Design review of the part built by this model. Coordinates are the model's own, in mm. A direction names the side the tool comes from. Coordinates: 2 decimals unless noted, no trailing zeros. Write each loop counter-clockwise with the first axis right and the second up, starting at its lowest first coordinate (ties: lowest second). Pieces come first, ordered by that corner, then holes.
Q1. For probe 1 along X at (y, z) = (10, 10.5); probe 2 along Y at (x, z) = (70, 4); probe 3 along Z at (x, y) = (27.5, -21.5), list the stretches that pass through material, from the lowest coordinate up.
Q2. Mouldability with a two-part tool opening along Y and no side actions: class faces 3 (the flat face through (-1, 22, -1)), 4 (the cylindrical face through (40, -20, 0)) as pulls with the +Y half, pulls with the -Y half, needs draft (parallel to the pull), parting line crosses it, or undercut.
Q3. Insertion check: pin 1 (0.5 mm diameter, centred on x = 27.5, y = -13, fed in from -Z); pin 2 (1.2 mm diameter, centred on x = 71, y = -13.5, fed in from +Z); pin 3 (5 mm diameter, centred on x = 45, y = -6.5, fed in from +Z); pin 4 (0.5 mm diameter, centred on x = 8, y = -13.5, fed in from +Z). Each pin has a flat end and moves straight along its axis. Give the tip position at first contact, or say it passes through.
Q4. Take a section at D-D (y = 14). Give the boundary of the cut face in (x, z).
Q5. Take a section at A-A (y = -3.5). Give the boundary of the cut face in (x, z).
Q6. Take a section at B-B (x = 5). State how many separate pieces and enclosed holes the cut face has, and give its area (3 significant figures).
Q7. Take a section at C-C (z = 22.5). Give the boundary of the cut face in (x, y).
Q8. Machinability: for faces 1 (the flat face through (30, -20, 4)), 2 (the flat face through (78.33, 23.87, 41.13)), which of the approach directions +Z, -Z, +X, -X, +Y, -Y give a long, thin tool a straight path to every point of the face, cutting with its end or side? Answer none if there is none.
```python
from build123d import *

# Parameters (mm, degrees)
BOSS_EXTRUDE1_DEPTH     = 80
CUT_EXTRUDE1_DEPTH      = 116.337274212
CUT_EXTRUDE1_DEPTH_BACK = 116.337274212
SKETCH2_W               = 76
SKETCH2_H               = 61.532163543
SKETCH3_W               = 18
SKETCH3_H               = 14.744736797
CUT_EXTRUDE2_DEPTH      = 20
BOSS_EXTRUDE2_DEPTH     = 1
BOSS_EXTRUDE3_START     = -81
BOSS_EXTRUDE3_DEPTH     = 1


with BuildPart() as part:
    # Sketch1 → Boss-Extrude1 (new body)
    with BuildSketch(Plane(origin=(0, 0, 0), x_dir=(0, 0, -1), z_dir=(1, 0, 0))):
        with BuildLine():
            Line((-17.20219293, -12.045105163), (-63.088307838, 53.48705838))
            Line((-63.088307838, 53.48705838), (-62.269155794, 54.060634816))
            Line((-62.269155794, 54.060634816), (-16.383040886, -11.471528727))
            ThreePointArc((-16.383040886, -11.471528727), (0, -20), (16.383040886, -11.471528727))
            Line((16.383040886, -11.471528727), (62.269155794, 54.060634816))
            Line((62.269155794, 54.060634816), (63.088307838, 53.48705838))
            Line((63.088307838, 53.48705838), (17.20219293, -12.045105163))
            ThreePointArc((17.20219293, -12.045105163), (0, -21), (-17.20219293, -12.045105163))
        make_face()
        with BuildLine():
            ThreePointArc((7.788873039, -19.5021398), (0, -21), (-7.788873039, -19.5021398))
            ThreePointArc((-7.788873039, -19.5021398), (-2.130530499, -24.056165822), (0, -31))
            ThreePointArc((0, -31), (2.130530499, -24.056165822), (7.788873039, -19.5021398))
        make_face()
    extrude(amount=BOSS_EXTRUDE1_DEPTH)

    # Sketch2 → Cut-Extrude1 (cut, two sides: drawn at the far end of the back side and taken through both)
    with BuildSketch(Plane.XY.offset(-CUT_EXTRUDE1_DEPTH_BACK)):
        with Locations((40, 20.720976608)):
            Rectangle(SKETCH2_W, SKETCH2_H)
    extrude(amount=CUT_EXTRUDE1_DEPTH + CUT_EXTRUDE1_DEPTH_BACK, mode=Mode.SUBTRACT)

    # Sketch3 → Cut-Extrude2 (cut)
    with BuildSketch(Plane(origin=(0, 0, 0), x_dir=(1, 0, 0), z_dir=(0, 1, 0))):
        with Locations((10, -8.191520442)):
            Rectangle(SKETCH3_W, SKETCH3_H)
        with Locations((10, 8.191520442)):
            Rectangle(SKETCH3_W, SKETCH3_H)
        with Locations((30, 8.191520442)):
            Rectangle(SKETCH3_W, SKETCH3_H)
        with Locations((30, -8.191520442)):
            Rectangle(SKETCH3_W, SKETCH3_H)
        with Locations((50, -8.191520442)):
            Rectangle(SKETCH3_W, SKETCH3_H)
        with Locations((50, 8.191520442)):
            Rectangle(SKETCH3_W, SKETCH3_H)
        with Locations((70, -8.191520442)):
            Rectangle(SKETCH3_W, SKETCH3_H)
        with Locations((70, 8.191520442)):
            Rectangle(SKETCH3_W, SKETCH3_H)
    extrude(amount=-CUT_EXTRUDE2_DEPTH, mode=Mode.SUBTRACT)

    # Sketch4 → Boss-Extrude2 (add)
    with BuildSketch(Plane(origin=(80, 0, 0), x_dir=(0, 0, -1), z_dir=(1, 0, 0))):
        with BuildLine():
            Line((-62.269155794, 54.060634816), (62.269155794, 54.060634816))
            Line((62.269155794, 54.060634816), (16.383040886, -11.471528727))
            ThreePointArc((16.383040886, -11.471528727), (0, -20), (-16.383040886, -11.471528727))
            Line((-16.383040886, -11.471528727), (-62.269155794, 54.060634816))
        make_face()
        with BuildLine():
            Line((-62.269155794, 54.060634816), (-63.088307838, 53.48705838))
            Line((-63.088307838, 53.48705838), (-17.20219293, -12.045105163))
            ThreePointArc((-17.20219293, -12.045105163), (-13.03994578, -16.460857026), (-7.788873039, -19.5021398))
            ThreePointArc((-7.788873039, -19.5021398), (-2.130530499, -24.056165822), (0, -31))
            ThreePointArc((0, -31), (2.130530499, -24.056165822), (7.788873039, -19.5021398))
            ThreePointArc((7.788873039, -19.5021398), (13.03994578, -16.460857026), (17.20219293, -12.045105163))
            Line((17.20219293, -12.045105163), (63.088307838, 53.48705838))
            Line((63.088307838, 53.48705838), (62.269155794, 54.060634816))
            Line((62.269155794, 54.060634816), (16.383040886, -11.471528727))
            ThreePointArc((16.383040886, -11.471528727), (0, -20), (-16.383040886, -11.471528727))
            Line((-16.383040886, -11.471528727), (-62.269155794, 54.060634816))
        make_face()
    extrude(amount=BOSS_EXTRUDE2_DEPTH)

    # Sketch4<3> → Boss-Extrude3 (add)
    with BuildSketch(Plane(origin=(80, 0, 0), x_dir=(0, 0, -1), z_dir=(1, 0, 0)).offset(BOSS_EXTRUDE3_START)):
        with BuildLine():
            Line((-62.269155794, 54.060634816), (62.269155794, 54.060634816))
            Line((62.269155794, 54.060634816), (16.383040886, -11.471528727))
            ThreePointArc((16.383040886, -11.471528727), (0, -20), (-16.383040886, -11.471528727))
            Line((-16.383040886, -11.471528727), (-62.269155794, 54.060634816))
        make_face()
        with BuildLine():
            Line((-62.269155794, 54.060634816), (-63.088307838, 53.48705838))
            Line((-63.088307838, 53.48705838), (-17.20219293, -12.045105163))
            ThreePointArc((-17.20219293, -12.045105163), (-13.03994578, -16.460857026), (-7.788873039, -19.5021398))
            ThreePointArc((-7.788873039, -19.5021398), (-2.130530499, -24.056165822), (0, -31))
            ThreePointArc((0, -31), (2.130530499, -24.056165822), (7.788873039, -19.5021398))
            ThreePointArc((7.788873039, -19.5021398), (13.03994578, -16.460857026), (17.20219293, -12.045105163))
            Line((17.20219293, -12.045105163), (63.088307838, 53.48705838))
            Line((63.088307838, 53.48705838), (62.269155794, 54.060634816))
            Line((62.269155794, 54.060634816), (16.383040886, -11.471528727))
            ThreePointArc((16.383040886, -11.471528727), (0, -20), (-16.383040886, -11.471528727))
            Line((-16.383040886, -11.471528727), (-62.269155794, 54.060634816))
        make_face()
    extrude(amount=BOSS_EXTRUDE3_DEPTH)


solid = part.part
```
Response:
1. probe 1: x = -1 to 0, 80 to 81
1. probe 2: y = -21.89 to -20
1. probe 3: z = -4.44 to 4.44
2. face 3: needs draft
2. face 4: pulls with the +Y half
3. pin 1: stops at z = -16.69
3. pin 2: stops at z = 16.57
3. pin 3: passes through
3. pin 4: stops at z = 16.29
4. outline: (-1, -35.44) - (2, -35.44) - (2, -34.22) - (0, -34.22) - (0, 34.22) - (2, 34.22) - (2, 35.44) - (-1, 35.44) - close; (78, -35.44) - (81, -35.44) - (81, 35.44) - (78, 35.44) - (78, 34.22) - (80, 34.22) - (80, -34.22) - (78, -34.22) - close
5. outline: (-1, -23.19) - (2, -23.19) - (2, -21.96) - (0, -21.96) - (0, 21.96) - (2, 21.96) - (2, 23.19) - (-1, 23.19) - close; (78, -23.19) - (81, -23.19) - (81, 23.19) - (78, 23.19) - (78, 21.96) - (80, 21.96) - (80, -21.96) - (78, -21.96) - close
6. separate pieces: 5
6. enclosed holes: 0
6. area: 56.0 mm2
7. outline: (-1, -4.48) - (2, -4.48) - (2, -2.74) - (0, -2.74) - (0, 54.06) - (-1, 54.06) - close; (78, -4.48) - (81, -4.48) - (81, 54.06) - (80, 54.06) - (80, -2.74) - (78, -2.74) - close
8. face 1: +Z, -Z, +Y
8. face 2: +Y
